Work out the finished part from the listing and answer in its coordinate system (mm). Round coordinates to 2 decimals unless told otherwise and drop trailing zeros. Write each loop counter-clockwise with the first axis right and the second up, starting at its lowest first coordinate (ties: lowest second). Pieces come first, ordered by that corner, then holes. Notation, with made-up numbers: (54.25, -18) - (89.25, -18) arc R25 ccw to (89.25, -4) - close; hole circle Ø7 at (-12.75, 45). An arc over 180 degrees is marked (long way). Answer as a JSON object with one key per item and string values.
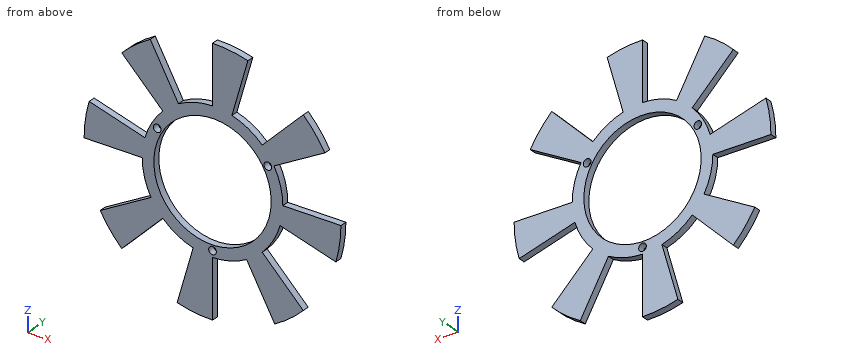
```python
from build123d import *

# Parameters (mm, degrees)
SKETCH1_R           = 30.25
SKETCH1_R_2         = 25.25
EXTRUDE_THIN1_DEPTH = 3
SKETCH2_R           = 1.65
CUT_EXTRUDE3_DEPTH  = 10
BOSS_EXTRUDE1_DEPTH = 3


with BuildPart() as part:
    # Sketch1 → Extrude-Thin1 (new body)
    with BuildSketch(Plane(origin=(0, 0, 0), x_dir=(1, 0, 0), z_dir=(0, 1, 0))):
        Circle(SKETCH1_R)
        Circle(SKETCH1_R_2, mode=Mode.SUBTRACT)
    extrude(amount=-EXTRUDE_THIN1_DEPTH)

    # Sketch2 → Cut-Extrude3 (cut)
    with BuildSketch(Plane(origin=(0, 0, 0), x_dir=(1, 0, 0), z_dir=(0, 1, 0))):
        with Locations((0, 27.5)):
            Circle(SKETCH2_R)
        with Locations((23.815698604, -13.75)):
            Circle(SKETCH2_R)
        with Locations((-23.815698604, -13.75)):
            Circle(SKETCH2_R)
    extrude(amount=-CUT_EXTRUDE3_DEPTH, mode=Mode.SUBTRACT)

    # Sketch5 → Boss-Extrude1 (add)
    with BuildSketch(Plane.XZ.offset(3)):
        with BuildLine():
            Line((0, 55.25), (0, 30.25))
            ThreePointArc((0, 30.25), (4.209986304, 29.955609079), (8.338030013, 29.078166302))
            Line((8.338030013, 29.078166302), (15.228963909, 53.109708701))
            ThreePointArc((15.228963909, 53.109708701), (7.689313828, 54.712310798), (0, 55.25))
        make_face()
        with BuildLine():
            Line((39.067649661, 39.067649661), (21.389980131, 21.389980131))
            ThreePointArc((21.389980131, 21.389980131), (24.158724179, 18.20490445), (26.457246141, 14.665491012))
            Line((26.457246141, 14.665491012), (48.322738819, 26.785731519))
            ThreePointArc((48.322738819, 26.785731519), (44.12461193, 33.250280029), (39.067649661, 39.067649661))
        make_face()
        with BuildLine():
            Line((55.25, 0), (30.25, 0))
            ThreePointArc((30.25, 0), (29.955609079, -4.209986304), (29.078166302, -8.338030013))
            Line((29.078166302, -8.338030013), (53.109708701, -15.228963909))
            ThreePointArc((53.109708701, -15.228963909), (54.712310798, -7.689313828), (55.25, 0))
        make_face()
        with BuildLine():
            Line((39.067649661, -39.067649661), (21.389980131, -21.389980131))
            ThreePointArc((21.389980131, -21.389980131), (18.20490445, -24.158724179), (14.665491012, -26.457246141))
            Line((14.665491012, -26.457246141), (26.785731519, -48.322738819))
            ThreePointArc((26.785731519, -48.322738819), (33.250280029, -44.12461193), (39.067649661, -39.067649661))
        make_face()
        with BuildLine():
            Line((0, -55.25), (0, -30.25))
            ThreePointArc((0, -30.25), (-4.209986304, -29.955609079), (-8.338030013, -29.078166302))
            Line((-8.338030013, -29.078166302), (-15.228963909, -53.109708701))
            ThreePointArc((-15.228963909, -53.109708701), (-7.689313828, -54.712310798), (0, -55.25))
        make_face()
        with BuildLine():
            Line((-39.067649661, -39.067649661), (-21.389980131, -21.389980131))
            ThreePointArc((-21.389980131, -21.389980131), (-24.158724179, -18.20490445), (-26.457246141, -14.665491012))
            Line((-26.457246141, -14.665491012), (-48.322738819, -26.785731519))
            ThreePointArc((-48.322738819, -26.785731519), (-44.12461193, -33.250280029), (-39.067649661, -39.067649661))
        make_face()
        with BuildLine():
            Line((-55.25, 0), (-30.25, 0))
            ThreePointArc((-30.25, 0), (-29.955609079, 4.209986304), (-29.078166302, 8.338030013))
            Line((-29.078166302, 8.338030013), (-53.109708701, 15.228963909))
            ThreePointArc((-53.109708701, 15.228963909), (-54.712310798, 7.689313828), (-55.25, 0))
        make_face()
        with BuildLine():
            Line((-39.067649661, 39.067649661), (-21.389980131, 21.389980131))
            ThreePointArc((-21.389980131, 21.389980131), (-18.20490445, 24.158724179), (-14.665491012, 26.457246141))
            Line((-14.665491012, 26.457246141), (-26.785731519, 48.322738819))
            ThreePointArc((-26.785731519, 48.322738819), (-33.250280029, 44.12461193), (-39.067649661, 39.067649661))
        make_face()
    extrude(amount=-BOSS_EXTRUDE1_DEPTH)


solid = part.part
```
Item 1: A cutting plane is placed at B-B (x = 17). Write down the section's boundary in (y, z), and give its area (3 significant figures).
Results found:
{"outline": "(-3, -30.67) - (0, -30.67) - (0, -18.67) - (-3, -18.67) - close; (-3, 18.67) - (0, 18.67) - (0, 25.02) - (-3, 25.02) - close", "area": "55.1 mm²"}
Item 2: A cutting plane is placed at C-C (y = -1.7). Give the number of separate pieces and of enclosed holes in the cut face, and give its area (3 significant figures).
Results found:
{"separate pieces": "1", "enclosed holes": "4", "area": "3,230 mm²"}
Item 3: A cutting plane is placed at A-A (z = -17). Write down the section's boundary in (x, y), and give its area (3 significant figures).
Results found:
{"outline": "(-30.67, -3) - (-18.67, -3) - (-18.67, 0) - (-30.67, 0) - close; (18.67, -3) - (25.02, -3) - (25.02, 0) - (18.67, 0) - close", "area": "55.1 mm²"}
Item 4: Each of these flat-tipped pins is pushed along its axis until it touches: P1, Ø2.5, axis at x = -23.82, z = 13.75, coming from the -Y side; P2, Ø1, axis at y = -1, z = -22, coming from the +X side; P3, Ø0.9, axis at y = -2, z = -46, coming from the +X side; P4, Ø0.9, axis at y = -2, z = 38.5, coming from the -X side. Where does it stop, or does it pass through?
Results found:
{"P1": "through", "P2": "x = 22.5", "P3": "x = 31.27", "P4": "x = -38.95"}
Item 5: Consider line 1 along X through (y, z) = (-0.2, 38.5); line 2 along Z through (x, y) = (36.5, -0.6); line 3 along Z through (x, y) = (-19, -2.8). Determine where each line is inside the solid, lowest interval first.
Results found:
{"line 1": "-38.5 to -21.34, 0 to 11.04, 38.5 to 39.63", "line 2": "-41.48 to -36.5, -10.47 to 0, 20.23 to 36.5", "line 3": "-23.54 to -16.63, 16.63 to 34.28"}
